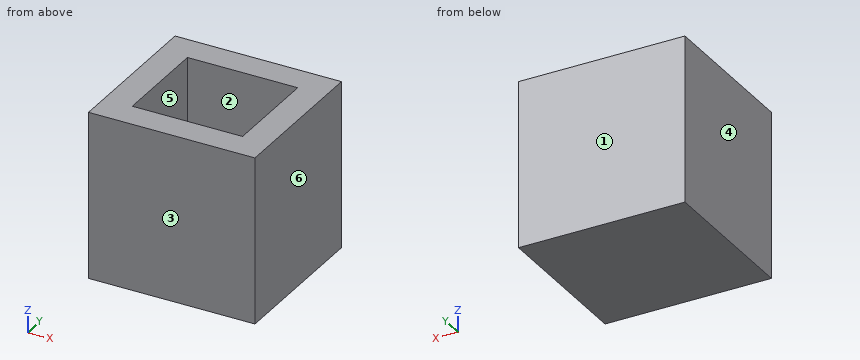
from build123d import *

# Parameters (mm, degrees)
F0_W     = 150.6082415581
F0_H     = 150.7464423776
F1_DEPTH = 140.462
F2_T     = -25.4
F3_DEPTH = 25.4


with BuildPart() as f1:
    # F0 (on Front) → F1 (new body)
    with BuildSketch(Plane.XZ):
        with Locations((0, -0.6814859807)):
            Rectangle(F0_W, F0_H)
    extrude(amount=F1_DEPTH)

    # F2
    f2_openings = [f1.faces().sort_by_distance(p)[0] for p in [
        (0, -70.231, 74.691735),
    ]]
    offset(amount=F2_T, openings=f2_openings)

    # F3 (add): a face of the model
    f3_faces = [f1.faces().sort_by_distance(p)[0] for p in [
        (0, -70.231, -50.6547071695),
    ]]
    extrude(f3_faces, amount=F3_DEPTH)


solid = f1.part
Check sheet for the modelled part. Datum: model origin and axes. Units: mm. Face numbers are marked on the shaded views. A direction names the side the tool comes from. Coordinates: 2 decimals unless noted, no trailing zeros. Write each loop counter-clockwise with the first axis right and the second up, starting at its lowest first coordinate (ties: lowest second). Pieces come first, ordered by that corner, then holes.
Item 1: Depth check by flat-ended pin: pin 1 Ø10 at (x, z) = (-58, 50.5) entering from +Y; pin 2 Ø12 at (x, y) = (19, -105.5) entering from +Z. Enter the tip coordinate at first touch or a pass-through.
Numbers:
pin 1: stops at y = 0
pin 2: stops at z = -25.25
Item 2: Access from +Z, -Z, +X, -X, +Y, -Y to the whole of each face (thin tool, end or side, straight path). Record for the marked faces 5 and 6.
Numbers:
face 5: +Z
face 6: +Z, -Z, +X, +Y, -Y
Item 3: Scan lines: probe 1 along X at (y, z) = (-57, 24); probe 2 along Y at (x, z) = (-32, 58); probe 3 along Z at (x, y) = (18.5, -98.5). Record each from-to range of solid material in increasing order.
Numbers:
probe 1: x = -75.3 to -49.9, 49.9 to 75.3
probe 2: y = -140.46 to -115.06, -25.4 to 0
probe 3: z = -76.05 to -25.25
Item 4: Cross-section at C-C on y = -74.5. Record the boundary of the cut face in (x, z), then the cut area to 3 significant figures.
Numbers:
outline: (-75.3, -76.05) - (75.3, -76.05) - (75.3, 74.69) - (49.9, 74.69) - (49.9, -25.25) - (-49.9, -25.25) - (-49.9, 74.69) - (-75.3, 74.69) - close
area: 12,700 mm2
Item 5: Mould release check, pull along Y, two halves, no side actions. Record for the marked faces 1, 2, 3 and 4: released by +Y, released by -Y, zero draft, split by the parting line, or undercut.
Numbers:
face 1: released by +Y
face 2: undercut
face 3: released by -Y
face 4: zero draft
Item 6: Cross-section at A-A on x = -14.5. Record the boundary of the cut face in (y, z).
Numbers:
outline: (-140.46, -76.05) - (0, -76.05) - (0, 74.69) - (-25.4, 74.69) - (-25.4, -25.25) - (-115.06, -25.25) - (-115.06, 74.69) - (-140.46, 74.69) - close
Item 7: Cross-section at B-B on z = 42.5. Record the boundary of the cut face in (x, y).
Numbers:
outline: (-75.3, -140.46) - (75.3, -140.46) - (75.3, 0) - (-75.3, 0) - close; hole (-49.9, -115.06) - (49.9, -115.06) - (49.9, -25.4) - (-49.9, -25.4) - close
